Input: part model. Units: mm. Frame: model coordinates. A direction names the side the tool comes from. Coordinates: 2 decimals unless noted, no trailing zeros. Write each loop counter-clockwise with the first axis right and the second up, starting at its lowest first coordinate (ties: lowest second). Pieces come first, ordered by that corner, then holes. Notation, with made-up numbers: (5.25, -4.5) -> (53.25, -4.5) arc R19 cw to (53.25, 12.5) -> close; hole circle Ø8 at (-39, 63). An arc over 180 degrees is marked (long way). Use one line per item in the form item = value. Start each with the question number.
(1) First-contact query: pin 1 (2 mm diameter, centred on y = -132.5, z = 39, fed in from -X) (3 decimals). Flat tip, straight axial feed; report the tip coordinate or a pass-through.
(2) Ray query, line 1 along Z through (x, y) = (20.5, -56) (3 decimals); line 2 along X through (y, z) = (-50.5, 9.5) (3 decimals). Return the intervals inside material, ascending.
(3) Cut plane B-B on x = -12.5. Return the cut outline in (y, z) (3 decimals), plus the area to 3 significant figures.
(4) Cut plane D-D on y = -169.5. Return the cut outline in (x, z) (3 decimals), plus the area to 3 significant figures.
(5) Cut plane A-A on z = -36.5. Return the cut outline in (x, y) (3 decimals), plus the area to 3 significant figures.
(6) Cut plane C-C on y = -124.5. Return the cut outline in (x, z) (3 decimals), plus the area to 3 significant figures.
(7) Set-up query: faces 1 (the face through (-50.8, -96, 1)), 2 (the face through (11, -112, -47.625)). Return all of +Z, -Z, +X, -X, +Y, -Y with unobstructed straight access to the full face (end or side cutting, diameter ignored); none if empty.
(8) Pull-direction query (Z, two-part tool) for faces 3 (the face through (10, -112, -50.8)), 4 (the face through (-47.625, -97, -1)), 5 (the face through (-4, -45.983, 48.681)); classes: released by +Z, released by -Z, zero draft, split by the parting line, or undercut.
```python
from build123d import *

# Parameters (mm, degrees)
F1_DEPTH      = 228.6
F3_DEPTH      = 50.801
F3_DEPTH_BACK = 50.801


with BuildPart() as f1:
    # F0 (on Front) → F1 (new body)
    with BuildSketch(Plane.XZ):
        with BuildLine():
            ThreePointArc((50.8, 47.625), (49.8700640303, 49.8700640303), (47.625, 50.8))
            Line((47.625, 50.8), (-47.625, 50.8))
            ThreePointArc((-47.625, 50.8), (-49.8700640303, 49.8700640303), (-50.8, 47.625))
            Line((-50.8, 47.625), (-50.8, -47.625))
            ThreePointArc((-50.8, -47.625), (-49.8700640303, -49.8700640303), (-47.625, -50.8))
            Line((-47.625, -50.8), (47.625, -50.8))
            ThreePointArc((47.625, -50.8), (49.8700640303, -49.8700640303), (50.8, -47.625))
            Line((50.8, -47.625), (50.8, 47.625))
        make_face()
        with BuildLine():
            Line((-44.45, 47.625), (44.45, 47.625))
            ThreePointArc((44.45, 47.625), (46.6950640303, 46.6950640303), (47.625, 44.45))
            Line((47.625, 44.45), (47.625, -44.45))
            ThreePointArc((47.625, -44.45), (46.6950640303, -46.6950640303), (44.45, -47.625))
            Line((44.45, -47.625), (-44.45, -47.625))
            ThreePointArc((-44.45, -47.625), (-46.6950640303, -46.6950640303), (-47.625, -44.45))
            Line((-47.625, -44.45), (-47.625, 44.45))
            ThreePointArc((-47.625, 44.45), (-46.6950640303, 46.6950640303), (-44.45, 47.625))
        make_face(mode=Mode.SUBTRACT)
    extrude(amount=F1_DEPTH)

    # F2 (on Top) → F3 (cut, two sides)
    with BuildSketch(Plane.XY) as f3_sk:
        Polygon((50.8, 0), (-50.8, 0), (-50.8, -85.2525225276), align=None)
        Polygon((-50.8, -107.5178349924), (-50.8, -228.6), (50.8, -228.6), align=None)
    extrude(amount=-F3_DEPTH, mode=Mode.SUBTRACT)
    extrude(f3_sk.sketch, amount=F3_DEPTH_BACK, mode=Mode.SUBTRACT)


solid = f1.part
```
Values:
q1.pin_1 = 47.625
q2.line_1 = -50.8 to -47.625, 47.625 to 50.8
q2.line_2 = 47.625 to 50.8
q3.outline = (-153.162, -50.8) -> (-53.115, -50.8) -> (-53.115, -47.625) -> (-153.162, -47.625) -> close; (-153.162, 47.625) -> (-53.115, 47.625) -> (-53.115, 50.8) -> (-153.162, 50.8) -> close
q3.area = 635 mm2
q4.outline = (1.209, -50.8) -> (47.625, -50.8) arc R3.175 ccw to (50.8, -47.625) -> (50.8, 47.625) arc R3.175 ccw to (47.625, 50.8) -> (1.209, 50.8) -> (1.209, 47.625) -> (44.45, 47.625) arc R3.175 cw to (47.625, 44.45) -> (47.625, -44.45) arc R3.175 cw to (44.45, -47.625) -> (1.209, -47.625) -> close
q4.area = 617 mm2
q5.outline = (-50.8, -107.518) -> (-47.625, -111.302) -> (-47.625, -82.588) -> (-50.8, -85.253) -> close; (47.625, -224.816) -> (50.8, -228.6) -> (50.8, 0) -> (47.625, -2.664) -> close
q5.area = 796 mm2
q6.outline = (-36.55, -50.8) -> (47.625, -50.8) arc R3.175 ccw to (50.8, -47.625) -> (50.8, 47.625) arc R3.175 ccw to (47.625, 50.8) -> (-36.55, 50.8) -> (-36.55, 47.625) -> (44.45, 47.625) arc R3.175 cw to (47.625, 44.45) -> (47.625, -44.45) arc R3.175 cw to (44.45, -47.625) -> (-36.55, -47.625) -> close
q6.area = 857 mm2
q7.face_1 = +Z, -Z, -X, +Y, -Y
q7.face_2 = +Y, -Y
q8.face_3 = released by -Z
q8.face_4 = undercut
q8.face_5 = zero draft
